from build123d import *

# Parameters (mm, degrees)
SKETCH1_R          = 23.6855
EXTRUDE1_DEPTH     = 82.423
CHAMFER1_SIZE      = 0.762
SKETCH6_R          = 17.4625
EXTRUDE2_DEPTH     = 5.969
SKETCH7_W          = 27.178
SKETCH7_H          = 10.31875
CUT_EXTRUDE4_DEPTH = 19.84248
HOLE1_D            = 4.7498
HOLE1_DEPTH        = 4.7498
CIRPATTERN1_COUNT  = 4
LPATTERN1_COUNT    = 2
LPATTERN1_PITCH    = 28.5496


with BuildPart() as part:
    # Sketch1 → Extrude1 (new body)
    with BuildSketch(Plane.XY):
        Circle(SKETCH1_R)
    extrude(amount=EXTRUDE1_DEPTH)

    # Sketch2 → Cut-Revolve1 (revolve, cut)
    with BuildSketch(Plane(origin=(0, 0, 0), x_dir=(1, 0, 0), z_dir=(0, 1, 0)), mode=Mode.PRIVATE) as cut_revolve1_sk:
        Polygon((23.6855, -82.423), (23.6855, -68.453), (22.4155, -69.723), (22.4155, -82.423), align=None)
    revolve(cut_revolve1_sk.sketch.rotate(Axis((0, 0, 0), (0, 0, 1)), 180), axis=Axis((0, 0, 0), (0, 0, 1)), mode=Mode.SUBTRACT)  # turned: the seam where the file's is

    # Sketch3 → Cut-Revolve2 (revolve, cut)
    with BuildSketch(Plane(origin=(0, 0, 0), x_dir=(1, 0, 0), z_dir=(0, 1, 0)), mode=Mode.PRIVATE) as cut_revolve2_sk:
        Polygon((22.4155, 0), (22.4155, -1.524), (23.6855, -2.794), (23.6855, 0), align=None)
    revolve(cut_revolve2_sk.sketch.rotate(Axis((0, 0, 0), (0, 0, -1)), 180), axis=Axis((0, 0, 0), (0, 0, -1)), mode=Mode.SUBTRACT)  # turned: the seam where the file's is

    # Chamfer1
    chamfer1_edges = [part.edges().sort_by_distance(p)[0] for p in [
        (22.4155, 0, 82.423),
    ]]
    chamfer(chamfer1_edges, length=CHAMFER1_SIZE)

    # S2D0002 → Cut-Revolve3 (revolve, cut)
    with BuildSketch(Plane(origin=(0, 0, 0), x_dir=(0, -1, 0), z_dir=(1, 0, 0)), mode=Mode.PRIVATE) as cut_revolve3_sk:
        Polygon((20.4597, -82.169), (23.7998, -82.169), (23.7998, -82.423), (14.2748, -82.423), (14.2748, -68.199), (19.2532, -68.199), (19.2532, -78.952393135), (19.917106865, -79.6163), align=None)
    cut_revolve3 = revolve(cut_revolve3_sk.sketch.rotate(Axis((0, -14.2748, 14.6685), (0, 0, -1)), 270), axis=Axis((0, -14.2748, 14.6685), (0, 0, -1)), mode=Mode.SUBTRACT)  # turned: the seam where the file's is

    # Sketch6 → Extrude2 (add)
    with BuildSketch(Plane(origin=(0, 0, 0), x_dir=(-1, 0, 0), z_dir=(0, 0, -1))):
        with Locations(Location((0, 0, 0), (0, 0, 180))):  # turned: the seam where the file's is
            Circle(SKETCH6_R)
    extrude(amount=EXTRUDE2_DEPTH)

    # Sketch7 → Revolve1 (revolve)
    with BuildSketch(Plane(origin=(0, 0, 0), x_dir=(0, 0, -1), z_dir=(1, 0, 0)), mode=Mode.PRIVATE) as revolve1_sk:
        with Locations((19.558, -5.159375)):
            Rectangle(SKETCH7_W, SKETCH7_H)
    revolve(revolve1_sk.sketch.rotate(Axis((0, 0, 0), (0, 0, -1)), 90), axis=Axis((0, 0, 0), (0, 0, -1)))  # turned: the seam where the file's is

    # S2D0001 → Cut-Revolve5 (revolve, cut)
    with BuildSketch(Plane(origin=(0, 0, 0), x_dir=(1, 0, 0), z_dir=(0, 1, 0))):
        Polygon((3.2639, 31.211260017), (3.2639, 18.2118), (0, 18.2118), (0, 33.147), (4.3815, 33.147), align=None)
    revolve(axis=Axis((0, 0, 31.308359971), (0, 0, -1)), mode=Mode.SUBTRACT)

    # Sketch9 → Cut-Revolve6 (revolve, cut)
    with BuildSketch(Plane(origin=(0, 0, 0), x_dir=(0, -1, 0), z_dir=(1, 0, 0)), mode=Mode.PRIVATE) as cut_revolve6_sk:
        with BuildLine():
            Line((-10.31875, 25.7302), (-10.033, 26.4922))
            Line((-10.033, 26.4922), (-10.033, 32.131))
            ThreePointArc((-10.033, 32.131), (-9.932678675, 32.674796865), (-9.644922533, 33.147))
            Line((-9.644922533, 33.147), (-10.31875, 33.147))
            Line((-10.31875, 33.147), (-10.31875, 25.7302))
        make_face()
    revolve(cut_revolve6_sk.sketch.rotate(Axis((0, 0, -12.65936), (0, 0, -1)), 90), axis=Axis((0, 0, -12.65936), (0, 0, -1)), mode=Mode.SUBTRACT)  # turned: the seam where the file's is

    # Sketch13 → Cut-Extrude4 (cut, symmetric)
    with BuildSketch(Plane(origin=(0, 0, 0), x_dir=(1, 0, 0), z_dir=(0, 1, 0))):
        Polygon((8.5852, 33.147), (8.5852, 28.194), (10.033, 26.7462), (10.033, 33.147), align=None)
        Polygon((-8.5852, 33.147), (-8.5852, 28.194), (-10.033, 26.7462), (-10.033, 33.147), align=None)
    extrude(amount=CUT_EXTRUDE4_DEPTH, both=True, mode=Mode.SUBTRACT)

    # Hole1
    with Locations(Plane(origin=(-15.850152054, 15.850152054, 76.073), x_dir=(0.707106781, 0.707106781, 0), z_dir=(-0.707106781, 0.707106781, 0))):
        with Locations((0, 0)):
            hole1 = Hole(HOLE1_D / 2, depth=HOLE1_DEPTH)

    # CirPattern1: Hole1 ×4 about axis
    cirpattern1_axis = Axis((0, 0, 0), (0, 0, 1))
    for i in range(1, CIRPATTERN1_COUNT):
        add(hole1.rotate(cirpattern1_axis, i * 360 / CIRPATTERN1_COUNT), mode=Mode.SUBTRACT)

    # LPattern1: Cut-Revolve3 ×2
    with Locations(*[(0, i * LPATTERN1_PITCH, 0) for i in range(1, LPATTERN1_COUNT)]):
        add(cut_revolve3, mode=Mode.SUBTRACT)


solid = part.part
Model file for the job. Use its own axes, mm. A direction names the side the tool comes from. Coordinates: 2 decimals unless noted, no trailing zeros. Write each loop counter-clockwise with the first axis right and the second up, starting at its lowest first coordinate (ties: lowest second). Pieces come first, ordered by that corner, then holes. Notation, with made-up numbers: (5, 38) - (13, 38) arc R13 ccw to (13, 53) - close; hole circle Ø4 at (71.5, 86). An arc over 180 degrees is marked (long way). Write each question's results on one line, items separated by ' | '. Start each with the question number.
1) Mould opens along X. For faces 5 (the face through (8, 8, -5.969)), 6 (the face through (-17.457, 16.008, 35.164)), 7 (the face through (-14.51, -13.78, 78.39)), 8 (the face through (-0.65, 9.34, 73.65)) say: pulls with the +X half, pulls with the -X half, needs draft (parallel to the pull), parting line crosses it, or undercut.
2) Cut at B-B (z = 72). Write the cut outline in (x, y).
3) Cut at C-C (z = 38.5). Write the cut outline in (x, y), then the cut area to 3 significant figures.
4) Probe line 1 along Y through (x, z) = (0, -24.25); line 2 along Z through (x, y) = (-8, -11.5); line 3 along Z through (x, y) = (-7, 20.5). List the from-to ranges inside material, lowest first. Write a range as from..to.
5) Flat gauge pins, fed straight in: P1, Ø1.5, axis at x = 10.5, y = -4.5, coming from the -Z side; P2, Ø5, axis at x = 1, y = 1, coming from the -Z side; P3, Ø1, axis at y = -18.5, z = 10, coming from the -X side. Where does each tip first touch, or does it go through?
6) Cut at A-A (z = -12). Write the cut outline in (x, y).
7) 3-axis set-ups, long thin cutter, end or side, ignore diameter. For faces 1 (the face through (0, 0, 82.423)), 2 (the face through (-0.708, 3.186, -24.621)), 3 (the face through (-12.515, -12.468, 76.04)), 4 (the face through (0, 14, 68.199)): which of +Z, -Z, +X, -X, +Y, -Y reach the whole face in a straight line?
Returned:
1) face 5: needs draft | face 6: parting line crosses it | face 7: undercut | face 8: undercut
2) outline: circle Ø44.83 at (0, 0); hole circle Ø9.96 at (0, -14.27); hole circle Ø9.96 at (0, 14.27)
3) outline: circle Ø47.37 at (0, 0) | area: 1,760 mm^2
4) line 1: -10.32..-3.26, 3.26..10.32 | line 2: -5.97..82.17 | line 3: 0..82.17
5) P1: z = -5.97 | P2: z = -32.34 | P3: x = -15.39
6) outline: circle Ø20.64 at (0, 0)
7) face 1: +Z, +X, -X, +Y, -Y | face 2: -Z | face 3: none | face 4: +Z
